from build123d import *

# Parameters (mm, degrees)
F0_W     = 90
F0_H     = 90
F1_DEPTH = 90
F3_W     = 30
F3_H     = 30
F4_DEPTH = 30
F2_W     = 30
F2_H     = 30
F5_DEPTH = 30


with BuildPart() as f1:
    # F0 (on Top) → F1 (new body)
    with BuildSketch(Plane.XY):
        Rectangle(F0_W, F0_H)
    extrude(amount=F1_DEPTH)

    # F3 (on face) → F4 (cut)
    with BuildSketch(Plane.XY.offset(90)):
        with Locations((-30, -30)):
            Rectangle(F3_W, F3_H)
        with Locations((-30, 30)):
            Rectangle(F3_W, F3_H)
        with Locations((30, 30)):
            Rectangle(F3_W, F3_H)
        with Locations((30, -30)):
            Rectangle(F3_W, F3_H)
    extrude(amount=-F4_DEPTH, mode=Mode.SUBTRACT)

    # F2 (on Top) → F5 (cut)
    with BuildSketch(Plane.XY):
        with Locations((30, 30)):
            Rectangle(F2_W, F2_H)
        with Locations((-30, 30)):
            Rectangle(F2_W, F2_H)
        with Locations((-30, -30)):
            Rectangle(F2_W, F2_H)
        with Locations((30, -30)):
            Rectangle(F2_W, F2_H)
    extrude(amount=F5_DEPTH, mode=Mode.SUBTRACT)


solid = f1.part
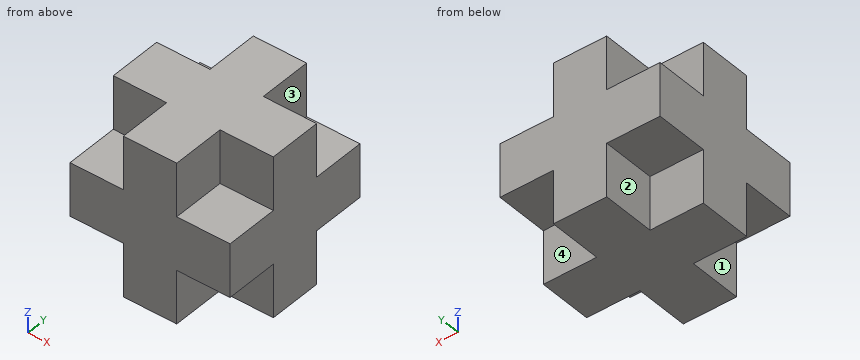
Verification items for the finished model (mm, model axes). Face numbers are marked on the shaded views. A direction names the side the tool comes from. Give positions to 0.01 mm unless a question says otherwise; leave off trailing zeros. Write each loop counter-clockwise with the first axis right and the second up, starting at its lowest first coordinate (ties: lowest second). Pieces come first, ordered by that corner, then holes.
(1) Cross-section at B-B (x = -34). Enter the section's corners in (y, z).
(2) Material ranges on line 1 (X direction, y = 32, z = 10.5); line 2 (Z direction, x = 27, y = -21.5), recorded low to high.
(3) Cross-section at A-A (z = 7.5). Enter the section's corners in (x, y), plus the area to 3 significant figures.
(4) Gauge pin test, flat ends, axial feed: pin 1 (15 mm diameter, centred on x = 26.5, y = 25, fed in from +Z); pin 2 (9 mm diameter, centred on x = 24.5, z = 13.5, fed in from -Y); pin 3 (1.5 mm diameter, centred on y = -17, z = 68.5, fed in from +X); pin 4 (1.5 mm diameter, centred on x = 30.5, y = 15.5, fed in from +Z). Record the tip position at first contact, or that the pin passes through.
(5) Access from +Z, -Z, +X, -X, +Y, -Y to the whole of each face (thin tool, end or side, straight path). Record for the marked faces 1, 2, 3 and 4.
Worked out:
1. outline: (-45, 30) - (-15, 30) - (-15, 0) - (15, 0) - (15, 30) - (45, 30) - (45, 60) - (15, 60) - (15, 90) - (-15, 90) - (-15, 60) - (-45, 60) - close
2. line 1: x = -15 to 15
2. line 2: z = 30 to 60
3. outline: (-45, -15) - (-15, -15) - (-15, -45) - (15, -45) - (15, -15) - (45, -15) - (45, 15) - (15, 15) - (15, 45) - (-15, 45) - (-15, 15) - (-45, 15) - close
3. area: 4,500 mm2
4. pin 1: stops at z = 60
4. pin 2: stops at y = -15
4. pin 3: stops at x = 15
4. pin 4: stops at z = 90
5. face 1: -Z, -X, -Y
5. face 2: -Z, -X, +Y
5. face 3: +Z, +X, +Y
5. face 4: -Z, +X, +Y
